Read the model definition and answer for the solid it produces. Units are mm, in the model's axes. A direction names the side the tool comes from. Give positions to 0.01 mm unless a question says otherwise; leave off trailing zeros. Write each loop counter-clockwise with the first axis right and the second up, starting at its lowest first coordinate (ties: lowest second). Pieces come first, ordered by that corner, then holes. Notation, with made-up numbers: (29.25, -35.5) -> (61.25, -35.5) arc R21 ccw to (61.25, -1.5) -> close; hole circle Ø8 at (12, -38). An arc over 180 degrees is marked (long way). Put each result on its own line as item: value. Start each with the question number.
from build123d import *

# Parameters (mm, degrees)
BOSS_EXTRUDE1_DEPTH      = 163
CUT_EXTRUDE2_DEPTH       = 187.46178402
BOSS_EXTRUDE2_DEPTH      = 3
FILLET5_R                = 10
BOSS_EXTRUDE3_DEPTH      = 10
BOSS_EXTRUDE3_DEPTH_BACK = 87.12
SKETCH14_R               = 4.9
SKETCH15_R               = 10.5
CUT_EXTRUDE6_DEPTH       = 10


with BuildPart() as part:
    # Sketch2 → Boss-Extrude1 (new body)
    with BuildSketch(Plane(origin=(0, 0, 0), x_dir=(1, 0, 0), z_dir=(0, 1, 0))):
        Polygon((-38.56, 47.45), (38.56, 47.45), (38.56, -47.45), (12.75, -47.45), (-38.56, -14.45), align=None)
    extrude(amount=-BOSS_EXTRUDE1_DEPTH)

    # Sketch4 → Cut-Extrude2 (cut, through all)
    with BuildSketch(Plane(origin=(38.56, 0, 0), x_dir=(0, 0, -1), z_dir=(1, 0, 0))):
        Polygon((47.45, 0), (27.45, 0), (47.45, -72.29), align=None)
    extrude(amount=-CUT_EXTRUDE2_DEPTH, mode=Mode.SUBTRACT)

    # Sketch13 → Boss-Extrude2 (add)
    with BuildSketch(Plane(origin=(0, -30.389847605, -66.576077827), x_dir=(-1, 0, 0), z_dir=(0, -0.41525187691718835, -0.909706479429905))):
        Polygon((38.56, -46.058979838), (27.805, -22.388979838), (-1.995, -22.388979838), (-12.75, -46.058979838), align=None)
    extrude(amount=-BOSS_EXTRUDE2_DEPTH)

    # Fillet5
    fillet5_edges = [part.edges().sort_by_distance(p)[0] for p in [
        (0, -163, -47.45),
        (0, 0, -27.45),
        (-27.805, -50.134369817, -55.914452207),
        (1.995, -50.134369817, -55.914452207),
    ]]
    fillet(fillet5_edges, radius=FILLET5_R)

    # Sketch14 → Boss-Extrude3 (add, two sides: drawn at the far end of the back side and taken through both)
    with BuildSketch(Plane(origin=(38.56, 0, 0), x_dir=(0, 0, -1), z_dir=(1, 0, 0)).offset(-BOSS_EXTRUDE3_DEPTH_BACK)):
        with Locations((-1.72, -131.263122253)):
            Circle(SKETCH14_R)
    extrude(amount=BOSS_EXTRUDE3_DEPTH + BOSS_EXTRUDE3_DEPTH_BACK)

    # Sketch15 → Cut-Extrude6 (cut)
    with BuildSketch(Plane(origin=(0, 0, -47.45), x_dir=(-1, 0, 0), z_dir=(0, 0, -1))):
        with Locations((0, -129.37)):
            Circle(SKETCH15_R)
    extrude(amount=-CUT_EXTRUDE6_DEPTH, mode=Mode.SUBTRACT)


solid = part.part
1) For a pull along X with two mould halves and no side action, classify faces 6 (the face through (38.56, -80, -1)), 7 (the face through (0.54, -39.36, -38.34)), 8 (the face through (2.28, -139.62, -42.52)), 9 (the face through (-38.56, -80, -16)) as pulls with the +X half, pulls with the -X half, needs draft (parallel to the pull), parting line crosses it, or undercut.
2) For faces 1 (the face through (26, -80, 47.45)), 2 (the face through (-12.569, -58.524, -50.436)), 3 (the face through (-43.63, -136.047, 2.782)), 4 (the face through (-1, -112, -47.45)), 5 (the face through (43.49, -136.047, 2.782)), determine the directions among +Z, -Z, +X, -X, +Y, -Y from which every point of the face is accessible in a straight line to the end or side of a thin tool.
3) A cutting plane is placed at B-B on z = 1.72. Give the vertices of the cut face in (x, y).
4) A cutting plane is placed at A-A on x = 16. Give the vertices of the cut face in (y, z), and give its area (3 significant figures).
5) A cutting plane is placed at C-C on y = -121.5. Give the vertices of the cut face in (x, z), and give its area (3 significant figures).
6) Straight lines are drawn through the part: line 1 (X direction, y = -129, z = -42); line 2 (X direction, y = -38, z = -12); line 3 (Z direction, x = 37.5, y = -107). For each, find the intervals that lie inside material, in ascending order. Write a range as [from, to].
7) Each of these flat-tipped pins is pushed along its axis until it touches: pin 1 Ø1 at (x, z) = (-9, -28) entering from +Y; pin 2 Ø6 at (x, y) = (-21, -39) entering from -Z; pin 3 Ø10 at (x, y) = (0, -142.5) entering from -Z. Where does it stop, or does it pass through?
8) A cutting plane is placed at D-D on x = 0. Give the vertices of the cut face in (y, z).
Results found:
1. face 6: pulls with the +X half
1. face 7: needs draft
1. face 8: undercut
1. face 9: pulls with the -X half
2. face 1: +Z, +X, -X, +Y, -Y
2. face 2: +X, -X, +Y
2. face 3: -X
2. face 4: -Z, +X, -X, -Y
2. face 5: +X
3. outline: (-48.56, -136.16) -> (-38.56, -136.16) -> (-38.56, -163) -> (38.56, -163) -> (38.56, -136.16) -> (48.56, -136.16) -> (48.56, -126.36) -> (38.56, -126.36) -> (38.56, 0) -> (-38.56, 0) -> (-38.56, -126.36) -> (-48.56, -126.36) -> close
4. outline: (-163, -37.45) arc R10 ccw to (-153, -47.45) -> (-72.29, -47.45) -> (-7.33, -29.48) arc R10 ccw to (0, -19.84) -> (0, 47.45) -> (-163, 47.45) -> close
4. area: 14,700 mm²
5. outline: (-38.56, -47.45) -> (-6.95, -47.45) -> (-6.95, -37.45) -> (6.95, -37.45) -> (6.95, -47.45) -> (38.56, -47.45) -> (38.56, 47.45) -> (12.75, 47.45) -> (-38.56, 14.45) -> close
5. area: 6,330 mm²
6. line 1: x = [-38.56, -10.49], [10.49, 38.56]
6. line 2: x = [-38.56, 38.56]
6. line 3: z = [-47.45, 47.45]
7. pin 1: stops at y = -3.57
7. pin 2: stops at z = -39.07
7. pin 3: stops at z = -47.45
8. outline: (-163, -37.45) arc R10 ccw to (-153, -47.45) -> (-139.87, -47.45) -> (-139.87, -37.45) -> (-118.87, -37.45) -> (-118.87, -47.45) -> (-72.29, -47.45) -> (-51.71, -56.85) -> (-50.46, -54.12) -> (-67.79, -46.21) -> (-7.33, -29.48) arc R10 ccw to (0, -19.84) -> (0, 39.25) -> (-163, 39.25) -> close
